Autodesk Inventor part; units mm, degrees
ref_plane "YZ Plane" through (0, 0, 0) normal (1, 0, 0) x (0, 1, 0)
ref_plane "XZ Plane" through (0, 0, 0) normal (0, 1, 0) x (-1, 0, 0)
ref_plane "XY Plane" through (0, 0, 0) normal (0, 0, 1) x (1, 0, 0)
sketch "Sketch1" plane through (0, 0, 0) normal (0, 1, 0) x (-1, 0, 0)
  arc A0 (97.7884, -35.051) -> (97.7884, 35.051) centre (106, 0) ccw
  arc A1 (75.9623, 44.4267) -> (97.7884, 35.051) centre (93.2264, 54.5237) ccw
  arc A2 (97.7884, -35.051) -> (75.9623, -44.4267) centre (93.2264, -54.5237) ccw
  arc A3 (-95.7901, 43.8265) -> (-95.7901, -43.8265) centre (-106, 0) ccw
  arc A4 (-95.7901, 43.8265) -> (-70.1803, 53.0916) centre (-90.1179, 68.1745) ccw
  arc A5 (-70.1803, -53.0916) -> (-95.7901, -43.8265) centre (-90.1179, -68.1745) ccw
  arc A6 (75.9623, 44.4267) -> (-70.1803, 53.0916) centre (0, 0) ccw
  arc A7 (-70.1803, -53.0916) -> (75.9623, -44.4267) centre (0, 0) ccw
  circle A8 centre (0, 0) radius 65
  circle A9 centre (-65, 0) radius 11.5
  circle A10 centre (-106, 0) radius 21.5
  arc A11 (0, 12.5) -> (0, -12.5) centre (0, 0) ccw
  arc A12 (106, -12.5) -> (106, 12.5) centre (106, 0) ccw
  line L0 (106, 12.5) -> (0, 12.5)
  line L1 (0, -12.5) -> (106, -12.5)
  line L2 (0, 0) -> (32.5, -56.2917)
  line L3 (-12.5, 0) -> (-53.5, 0)
  line L4 (0, 0) -> (23.2902, 40.3398)
  line L5 (23.2902, 40.3398) -> (32.5, 56.2917)
  circle A13 centre (32.5, 56.2917) radius 12.5
  circle A14 centre (32.5, -56.2917) radius 12.5
  dimension "d13" = 23
  dimension "d1" = 72
  dimension "d2" = 106
  dimension "d3" = 40
  dimension "d4" = 0
  dimension "d5" = 40
  dimension "d7" = 90
  dimension "d8" = 212
  dimension "d9" = 50
  dimension "d10" = 50
  dimension "d11" = 0
  dimension "d12" = 130
  dimension "d14" = 43
  dimension "d15" = 25
  dimension "d16" = 25
  dimension "d18" = 120
  dimension "d19" = 120
  dimension "d20" = 25
  dimension "d21" = 25
extrude "Extrusion1" add sketch "Sketch1" along normal blind 10 contours A2 A7 A5 A3 A4 A6 A1 A0 | L0 L4 L5 A13 A8 | A8 A14 L2 L1 | L0 A11 L3 A9 A8 A13 L5 L4 | L2 A14 A8 A9 L3 A11 L1
equation "\"d5\" = d3"
equation "\"d10\" = d9"
Part model, mm, in its own coordinate system. A direction names the side the tool comes from. Round coordinates to 2 decimals unless told otherwise and drop trailing zeros. Loops run counter-clockwise (first coordinate to the right, second up) from the corner with the lowest first, then second, coordinate; pieces in that order, holes last. Notation, with made-up numbers: (11.5, 16.5) -> (19.5, 16.5) arc R6 cw to (19.5, 24.5) -> close; hole circle Ø3 at (27.5, -27.5). An arc over 180 degrees is marked (long way). Use one line per item in the form item = value. Start each with the question number.
Item 1: Band-saw the part on C-C (z = 66). List the corners of the cut face in (x, y).
Item 2: Band-saw the part on B-B (z = 0). List the corners of the cut face in (x, y).
Item 3: Drill centre lines: line 1 along Z through (x, y) = (106, 7.75); line 2 along X through (y, z) = (1.5, -58); line 3 along X through (y, z) = (9.25, 19.5). Where is each one in solid material? Low to high.
Item 4: Tool access for faces 1 (the cylindrical face through (81.424, 4.93, 44.735)), 2 (the flat face through (-52, 5, -12.5)): list every direction of +Z, -Z, +X, -X, +Y, -Y with a clear straight run to the whole face (end or side of a thin tool).
Item 5: Band-saw the part on A-A (x = 106). List the corners of the cut face in (y, z), plus the area to 3 significant figures.
Item 6: Band-saw the part on D-D (x = -32.5). List the corners of the cut face in (y, z).
Item 7: Two-plate mould, pull along X, no slides. Class faces 3 (the cylindrical face through (-4, 4.93, 87.91)), 4 (the cylindrical face through (-85.497, 4.93, 36.078)), 5 (the flat face through (7, 0, -18)): released by +X, released by -X, zero draft, split by the parting line, or undercut.
Item 8: Drop flat-ended pins along their axis: pin 1 Ø1.5 at (x, y) = (121.5, 1.5) entering from -Z; pin 2 Ø6 at (x, y) = (22.5, 4.5) entering from +Z; pin 3 Ø1 at (x, y) = (92, 4) entering from +Z. Give the stop position or say it passes through.
Data:
q1.outline = (-58.21, 0) -> (-40.37, 0) -> (-40.37, 10) -> (-58.21, 10) -> close; (-24.63, 0) -> (58.21, 0) -> (58.21, 10) -> (-24.63, 10) -> close
q2.outline = (-142, 0) -> (-118.5, 0) -> (-118.5, 10) -> (-142, 10) -> close; (12.5, 0) -> (53.5, 0) -> (53.5, 10) -> (12.5, 10) -> close; (76.5, 0) -> (84.5, 0) -> (84.5, 10) -> (76.5, 10) -> close; (127.5, 0) -> (151, 0) -> (151, 10) -> (127.5, 10) -> close
q3.line_1 = -45 to -21.5, 21.5 to 45
q3.line_2 = -66.18 to -44.88, -20.12 to 66.18
q3.line_3 = -136.26 to 96.94, 115.06 to 146.56
q4.face_1 = +Z, +Y, -Y
q4.face_2 = +Y, -Y
q5.outline = (0, -45) -> (10, -45) -> (10, -21.5) -> (0, -21.5) -> close; (0, 21.5) -> (10, 21.5) -> (10, 45) -> (0, 45) -> close
q5.area = 470 mm^2
q6.outline = (0, -81.78) -> (10, -81.78) -> (10, -68.79) -> (0, -68.79) -> close; (0, -43.79) -> (10, -43.79) -> (10, -12.5) -> (0, -12.5) -> close; (0, 12.5) -> (10, 12.5) -> (10, 43.79) -> (0, 43.79) -> close; (0, 68.79) -> (10, 68.79) -> (10, 81.78) -> (0, 81.78) -> close
q7.face_3 = split by the parting line
q7.face_4 = undercut
q7.face_5 = zero draft
q8.pin_1 = -42.51
q8.pin_2 = 85.81
q8.pin_3 = 43.29
